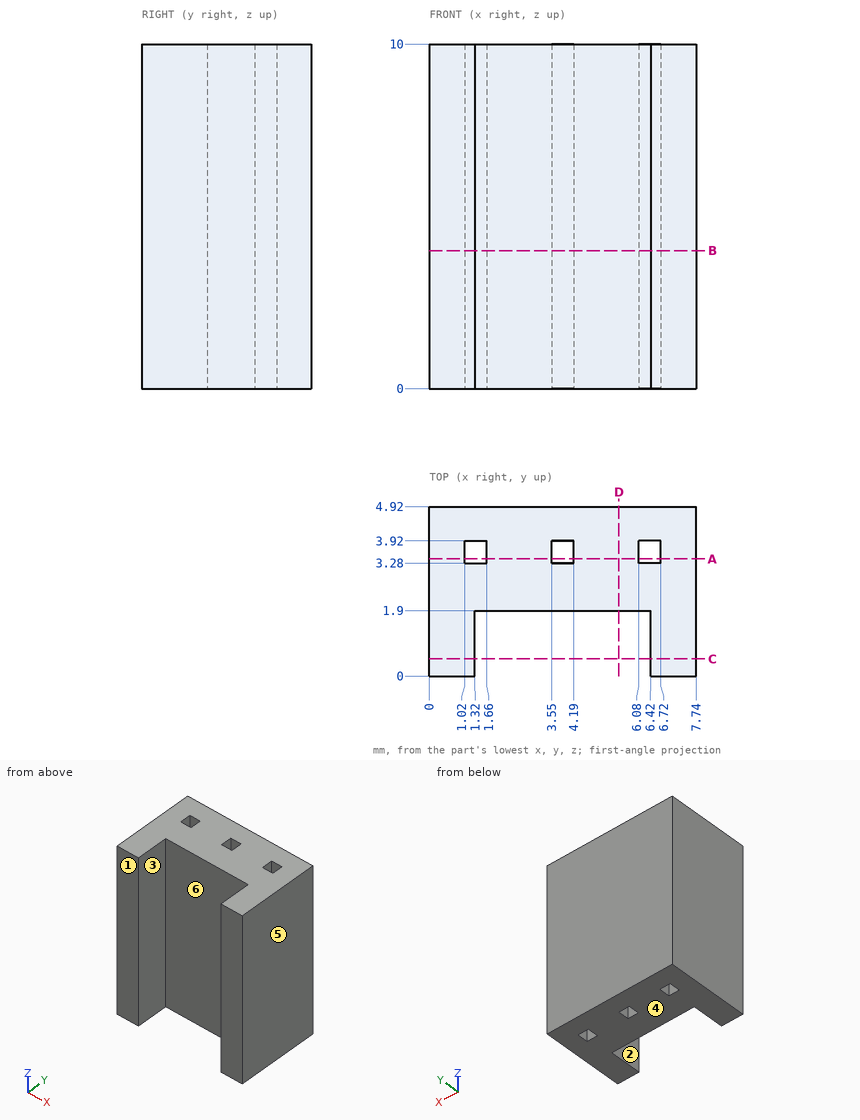
Geometry: see drawing. Coordinates: mm, zero at the bounding-box minimum. A direction names the side the tool comes from. Round coordinates to 2 decimals unless told otherwise and drop trailing zeros. Write each loop counter-clockwise with the first axis right and the second up, starting at its lowest first coordinate (ties: lowest second). Pieces come first, ordered by that corner, then holes.
Item 1: Set-up query: the marked faces 1 and 2. Return all of +Z, -Z, +X, -X, +Y, -Y with unobstructed straight access to the full face (end or side cutting, diameter ignored); none if empty.
Item 2: Pin query (flat end, axial travel): P1, Ø1.5, axis at x = 4, y = 4.5, coming from the -Z side; P2, Ø0.5, axis at x = 4, z = 3, coming from the -Y side. Return the tip coordinate at first contact, or that it passes through.
Item 3: Mould query, pull axis X, two halves, no side actions, for the marked faces 3, 4, 5 and 6. Classes: +X half, -X half, draft (parallel to the pull), parting line (faces both ways), or undercut.
Item 4: Section query B-B (z = 4). Return loops of the section in (x, y), plus the area to 3 significant figures.
Item 5: Section query A-A (y = 3.4). Return loops of the section in (x, z), plus the area to 3 significant figures.
Item 6: Section query D-D (x = 5.5). Return loops of the section in (y, z), plus the area to 3 significant figures.
Item 7: Section query C-C (y = 0.5). Return loops of the section in (x, z).
Item 8: Material intervals for L1, parallel to X at y = 0.85, z = 4; L2, parallel to X at y = 3.7, z = 1; L3, parallel to Y at x = 4.5, z = 6.5, sorted ascending.
Completed:
1. face 1: +Z, -Z, +X, -X, -Y
1. face 2: +Z, -Z, -Y
2. P1: stops at z = 0
2. P2: stops at y = 1.9
3. face 3: undercut
3. face 4: draft
3. face 5: +X half
3. face 6: undercut
4. outline: (0, 0) - (1.32, 0) - (1.32, 1.9) - (6.42, 1.9) - (6.42, 0) - (7.74, 0) - (7.74, 4.92) - (0, 4.92) - close; hole (1.02, 3.28) - (1.66, 3.28) - (1.66, 3.92) - (1.02, 3.92) - close; hole (3.55, 3.28) - (4.19, 3.28) - (4.19, 3.92) - (3.55, 3.92) - close; hole (6.08, 3.28) - (6.72, 3.28) - (6.72, 3.92) - (6.08, 3.92) - close
4. area: 27.2 mm2
5. outline: (0, 0) - (1.02, 0) - (1.02, 10) - (0, 10) - close; (1.66, 0) - (3.55, 0) - (3.55, 10) - (1.66, 10) - close; (4.19, 0) - (6.08, 0) - (6.08, 10) - (4.19, 10) - close; (6.72, 0) - (7.74, 0) - (7.74, 10) - (6.72, 10) - close
5. area: 58.2 mm2
6. outline: (1.9, 0) - (4.92, 0) - (4.92, 10) - (1.9, 10) - close
6. area: 30.2 mm2
7. outline: (0, 0) - (1.32, 0) - (1.32, 10) - (0, 10) - close; (6.42, 0) - (7.74, 0) - (7.74, 10) - (6.42, 10) - close
8. L1: x = 0 to 1.32, 6.42 to 7.74
8. L2: x = 0 to 1.02, 1.66 to 3.55, 4.19 to 6.08, 6.72 to 7.74
8. L3: y = 1.9 to 4.92
